The model under review builds one solid part; all positions refer to its coordinate system, in mm. A direction names the side the tool comes from. Coordinates: 2 decimals unless noted, no trailing zeros. Loops run counter-clockwise (first coordinate to the right, second up) from the corner with the lowest first, then second, coordinate; pieces in that order, holes last. Notation, with made-up numbers: M 48,-21.5 L 87,-21.5 A16 cw 87,-6.5 Z; hole C 63.5,36.5 d6. An arc over 180 degrees is marked long. Write item = value, one per line. Start each with the question number.
Q1. For faces 5 (the face through (24, 28, 81.788)), 6 (the face through (-0.54, 25.3, 5.82)), 7 (the face through (-9.144, 14, 88)), 8 (the face through (-91, 25.654, 0)), list the 3-axis set-ups (+Z, -Z, +X, -X, +Y, -Y) from which the entire face can be reached by the end or side of a thin tool; tool diameter is ignored.
Q2. Mouldability with a two-part tool opening along Y and no side actions: class faces 1 (the face through (-23.54, 27.3, 87.97)), 2 (the face through (-91, 14.986, 0)), 3 (the face through (-87.122, 20, 0)), 4 (the face through (-24, 9, 93.98)) as released by +Y, released by -Y, zero draft, split by the parting line, or undercut.
Q3. We need section C-C on y = 6. Give the boundary of the cut face in (x, z).
Q4. We need section A-A on x = -19. Give the boundary of the cut face in (y, z), and give its area (3 significant figures).
Q5. Wall thickness on probe 1 along Z at (x, y) = (17, 23.5); probe 2 along X at (y, z) = (35.5, -3); probe 3 along X at (y, z) = (5, 38): over which ranges is each line inside the solid? List them lowest first.
Q6. We need section D-D on x = 2. Give the boundary of the cut face in (y, z).
Q7. Clearance check with flat-ended pins moving along their axes: pin 1 Ø5 at (x, y) = (-28.5, 23) entering from -Z; pin 2 Ø5 at (x, z) = (40.5, 72) entering from +Y; pin 3 Ø5.5 at (x, y) = (-3, 10.5) entering from +Z. State where each tip first meets the part, or that it passes through.
Q8. We need section B-B on y = 34. Give the boundary of the cut face in (x, z).
from build123d import *

# Parameters (mm, degrees)
SKETCH2_W               = 81.788
SKETCH2_H               = 18.288
BOSS_EXTRUDE1_DEPTH     = 38.354
SKETCH3_R               = 20.32
BOSS_EXTRUDE2_DEPTH     = 9.144
BOSS_EXTRUDE3_START     = 9.144
BOSS_EXTRUDE3_DEPTH     = 8.128
BOSS_EXTRUDE4_START     = -76.708
SKETCH3_4_R             = 20.32
BOSS_EXTRUDE4_DEPTH     = 56.896
CUT_EXTRUDE1_DEPTH      = 8.128
SKETCH5_W               = 18.288
SKETCH5_H               = 12.192
CUT_EXTRUDE3_DEPTH      = 23.352
CUT_EXTRUDE3_DEPTH_BACK = 19.288


with BuildPart() as part:
    # Sketch2 → Boss-Extrude1 (new body, symmetric)
    with BuildSketch(Plane(origin=(0, 0, 0), x_dir=(0, 0, -1), z_dir=(1, 0, 0))):
        with Locations((-40.894, 9.144)):
            Rectangle(SKETCH2_W, SKETCH2_H)
        Polygon((-81.788, 36.576), (-81.788, 18.288), (-81.788, 0), (-93.98, 0), (-93.98, 18.288), align=None)
        with BuildLine():
            Line((0, 18.288), (0, 0))
            ThreePointArc((0, 0), (20.285688823, 21.500351201), (-2.356716256, 40.502871166))
            ThreePointArc((-2.356716256, 40.502871166), (-2.037100365, 38.550986103), (-1.930144722, 36.576))
            ThreePointArc((-1.930144722, 36.576), (-7.286575908, 23.644431186), (-20.218144722, 18.288))
            Line((-20.218144722, 18.288), (0, 18.288))
        make_face()
    extrude(amount=BOSS_EXTRUDE1_DEPTH, both=True)

    # Sketch3 → Boss-Extrude2 (add)
    with BuildSketch(Plane(origin=(38.354, 0, 0), x_dir=(0, 0, -1), z_dir=(1, 0, 0))):
        with Locations((0, 20.32)):
            Circle(SKETCH3_R)
    extrude(amount=BOSS_EXTRUDE2_DEPTH)

    # Sketch3<3> → Boss-Extrude3 (add)
    with BuildSketch(Plane(origin=(38.354, 0, 0), x_dir=(0, 0, -1), z_dir=(1, 0, 0)).offset(BOSS_EXTRUDE3_START)):
        with BuildLine():
            Line((-2.286, 10.420514963), (-2.286, 30.219485037))
            ThreePointArc((-2.286, 30.219485037), (-2.727219055, 30.107128089), (-3.162961291, 29.975116564))
            ThreePointArc((-3.162961291, 29.975116564), (-5.965678902, 25.116586312), (-10.109072361, 21.336))
            ThreePointArc((-10.109072361, 21.336), (-8.258111655, 14.401453566), (-2.286, 10.420514963))
        make_face()
        with BuildLine():
            ThreePointArc((10.16, 20.32), (7.951457728, 26.644548996), (2.286, 30.219485037))
            Line((2.286, 30.219485037), (2.286, 10.420514963))
            ThreePointArc((2.286, 10.420514963), (7.951457728, 13.995451004), (10.16, 20.32))
        make_face()
        with BuildLine():
            ThreePointArc((-10.109072361, 21.336), (-5.965678902, 25.116586312), (-3.162961291, 29.975116564))
            ThreePointArc((-3.162961291, 29.975116564), (-7.918036566, 26.686340938), (-10.109072361, 21.336))
        make_face()
    extrude(amount=BOSS_EXTRUDE3_DEPTH)

    # Sketch3<4> → Boss-Extrude4 (add)
    with BuildSketch(Plane(origin=(38.354, 0, 0), x_dir=(0, 0, -1), z_dir=(1, 0, 0)).offset(BOSS_EXTRUDE4_START)):
        with Locations((0, 20.32)):
            Circle(SKETCH3_4_R)
    extrude(amount=-BOSS_EXTRUDE4_DEPTH)

    # Sketch4 → Cut-Extrude1 (cut)
    with BuildSketch(Plane.ZY.offset(95.25)):
        with BuildLine():
            Line((19.607418086, 25.654), (-19.607418086, 25.654))
            ThreePointArc((-19.607418086, 25.654), (-20.32, 20.32), (-19.607418086, 14.986))
            Line((-19.607418086, 14.986), (19.607418086, 14.986))
            ThreePointArc((19.607418086, 14.986), (20.141066699, 17.629306363), (20.32, 20.32))
            ThreePointArc((20.32, 20.32), (20.141066699, 23.010693637), (19.607418086, 25.654))
        make_face()
    extrude(amount=-CUT_EXTRUDE1_DEPTH, mode=Mode.SUBTRACT)

    # Sketch5 → Cut-Extrude3 (cut, two sides)
    with BuildSketch(Plane(origin=(0, 18.288, 0), x_dir=(1, 0, 0), z_dir=(0, 1, 0))) as cut_extrude3_sk:
        with Locations((0, -87.884)):
            Rectangle(SKETCH5_W, SKETCH5_H)
    extrude(amount=CUT_EXTRUDE3_DEPTH, mode=Mode.SUBTRACT)
    extrude(cut_extrude3_sk.sketch, amount=-CUT_EXTRUDE3_DEPTH_BACK, mode=Mode.SUBTRACT)


solid = part.part
Returned:
q1.face_5 = +X, -X, +Y
q1.face_6 = none
q1.face_7 = +Z, +Y, -Y
q1.face_8 = +Z, -Z, -X
q2.face_1 = released by +Y
q2.face_2 = undercut
q2.face_3 = undercut
q2.face_4 = zero draft
q3.outline = M -95.25,-14.42 L 47.5,-14.42 L 47.5,14.42 L 38.35,14.42 L 38.35,93.98 L 9.14,93.98 L 9.14,81.79 L -9.14,81.79 L -9.14,93.98 L -38.35,93.98 L -38.35,14.42 L -95.25,14.42 Z
q4.outline = M 0,0 A20.32 ccw long 40.5,2.36 A18.29 cw 18.29,20.22 L 18.29,81.79 L 36.58,81.79 L 18.29,93.98 L 0,93.98 Z
q4.area = 2,590 mm^2
q5.probe_1 = -20.07 to 7.43, 81.79 to 90.51
q5.probe_2 = -95.25 to 47.5
q5.probe_3 = -38.35 to 38.35
q6.outline = M 0,0 A20.32 ccw long 40.5,2.36 A18.29 cw 18.29,20.22 L 18.29,81.79 L 0,81.79 Z
q7.pin_1 = -20.32
q7.pin_2 = 18.29
q7.pin_3 = 81.79
q8.outline = M -95.25,-15.03 L 47.5,-15.03 L 47.5,15.03 L 38.35,15.03 L 38.35,2.11 L -38.35,2.11 L -38.35,15.03 L -95.25,15.03 Z; M -38.35,81.79 L -9.14,81.79 L -9.14,83.51 L -38.35,83.51 Z; M 9.14,81.79 L 38.35,81.79 L 38.35,83.51 L 9.14,83.51 Z
